For this review, use the dimensioned drawing (mm, ordinates from the lowest corner) and the shaded views. A direction names the side the tool comes from. Give positions to 0.01 mm unless a question says otherwise; leave off trailing zeros. Write each loop counter-clockwise with the first axis right and the second up, starting at its lowest first coordinate (ties: lowest second). Pieces come first, ordered by that corner, then holes. Notation, with made-up numbers: (0, -4.75) -> (20, -4.75) arc R19 ccw to (20, 32.25) -> close; hole circle Ø10 at (23.5, -34). An arc over 180 degrees is marked (long way). Return JSON: item names as keys, results as strings.
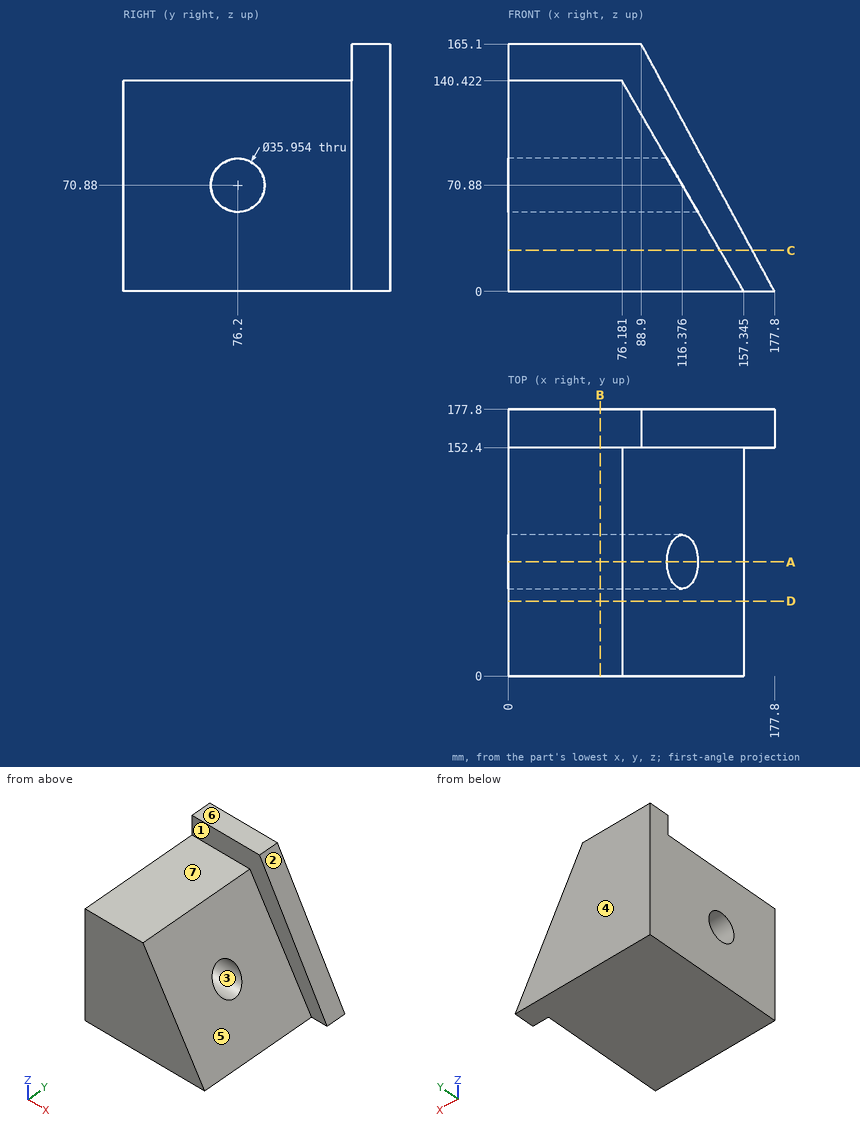
1. Add section C-C, the plane z = 27.5. State the section outline as (x, y) points.
Results found:
{"outline": "(0, 0) -> (141.45, 0) -> (141.45, 152.4) -> (162.99, 152.4) -> (162.99, 177.8) -> (0, 177.8) -> close"}
2. Add section A-A, the plane y = 76.2. State the section outline as (x, z) points (1 decimal), plus the area to 3 significant figures.
Results found:
{"outline": "(0, 0) -> (157.3, 0) -> (126.8, 52.9) -> (0, 52.9) -> close; (0, 88.9) -> (106, 88.9) -> (76.2, 140.4) -> (0, 140.4) -> close", "area": "12,200 mm²"}
3. The part is to be moulded in two halves that separate along Y. For the marked faces 1, 2, 3 and 4, say which applies: +Y half, -Y half, draft (parallel to the pull), parting line (faces both ways), or undercut.
Results found:
{"face 1": "-Y half", "face 2": "draft", "face 3": "undercut", "face 4": "+Y half"}
4. To check wall thickness, follow probe 1 along Z at (x, y) = (55, 76.2); probe 2 along Y at (x, z) = (109.5, 72); probe 3 along Z at (x, y) = (21, 117). State the ranges of each line that lie inside material, in increasing order.
Results found:
{"probe 1": "z = 0 to 52.9, 88.86 to 140.42", "probe 2": "y = 0 to 58.26, 94.14 to 177.8", "probe 3": "z = 0 to 140.42"}
5. Add section B-B, the plane x = 61.5. State the section outline as (y, z) points.
Results found:
{"outline": "(0, 0) -> (177.8, 0) -> (177.8, 165.1) -> (152.4, 165.1) -> (152.4, 140.42) -> (0, 140.42) -> close; hole circle Ø35.95 at (76.2, 70.88)"}
6. For pin 1 (3 mm diameter, centred on x = 119.5, y = 127.5, fed in from -Z); pin 2 (1 mm diameter, centred on x = 38, y = 107, fed in from +Z); pin 3 (1.5 mm diameter, centred on y = 157, z = 49, fed in from +X); pin 4 (1.5 mm diameter, centred on x = 144, y = 68, fed in from +Z) (1 decimal), all flat-tipped, find the tip position at first contact; note any pin that passes through.
Results found:
{"pin 1": "stops at z = 0", "pin 2": "stops at z = 140.42", "pin 3": "stops at x = 151.82", "pin 4": "stops at z = 24.4"}
7. Add section D-D, the plane y = 50. State the section outline as (x, z) points (1 decimal), plus the area to 3 significant figures.
Results found:
{"outline": "(0, 0) -> (157.3, 0) -> (76.2, 140.4) -> (0, 140.4) -> close", "area": "16,400 mm²"}
8. For the marked faces 5, 6 and 7, list the 3-axis set-ups (+Z, -Z, +X, -X, +Y, -Y) from which the entire face can be reached by the end or side of a thin tool; tool diameter is ignored.
Results found:
{"face 5": "+Z, +X, -Y", "face 6": "+Z, +X, -X, +Y, -Y", "face 7": "+Z, +X, -X, -Y"}
